For this review, take the finished solid that the model builds, in its own axes (mm). A direction names the side the tool comes from. Round coordinates to 2 decimals unless told otherwise and drop trailing zeros. Loops run counter-clockwise (first coordinate to the right, second up) from the corner with the lowest first, then second, coordinate; pieces in that order, holes last. Notation, with made-up numbers: (19.5, -37) -> (46.5, -37) arc R28 ccw to (46.5, -6) -> close; hole circle Ø7 at (88, -18.75). An arc over 180 degrees is marked (long way). One line per question, with ' | ' between items. Start each with the question number.
1. Consider section D-D (y = 8.5). Write out the cut boundary in (x, z).
2. For faces 1 (the face through (12.52, 11.04, 26.51)), 2 (the face through (13, 10, 60.198)), list the 3-axis set-ups (+Z, -Z, +X, -X, +Y, -Y) from which the entire face can be reached by the end or side of a thin tool; tool diameter is ignored.
3. Consider section C-C (y = 4). Write out the cut boundary in (x, z), and give its area (3 significant figures).
4. Wall thickness on line 1 along Z through (x, y) = (13.75, 13); line 2 along Z through (x, y) = (12, 7.25); line 3 along Z through (x, y) = (20.25, 16.5): over which ranges is each line inside the solid? List them lowest first.
5. Consider section B-B (x = 21). Write out the cut boundary in (y, z) (3 decimals).
6. Consider section A-A (z = 63.5). Write out the cut boundary in (x, y), and give its area (3 significant figures).
7. Draft analysis for pull direction X (two halves, no side actions). For faces 3 (the face through (25.4, 9, 38)), 4 (the face through (3.05, 9.66, 38.03)), 5 (the face through (12.522, 10.478, 49.364)), 6 (the face through (22.35, 9.66, 63.57)), state which applies: pulls with the +X half, pulls with the -X half, needs draft (parallel to the pull), parting line crosses it, or undercut.
Autodesk Inventor part; units mm, degrees
ref_plane "YZ Plane" through (0, 0, 0) normal (1, 0, 0) x (0, 1, 0)
ref_plane "XZ Plane" through (0, 0, 0) normal (0, 1, 0) x (-1, 0, 0)
ref_plane "XY Plane" through (0, 0, 0) normal (0, 0, 1) x (1, 0, 0)
sketch "Sketch1" plane through (0, 0, 0) normal (0, 0, 1) x (1, 0, 0)
  line L0 (0, 0) -> (25.4, 0)
  line L1 (25.4, 0) -> (25.4, 19.05)
  line L2 (25.4, 19.05) -> (0, 19.05)
  line L3 (0, 19.05) -> (0, 0)
  dimension "d0" = 25.4
  dimension "d1" = 19.05
extrude "Stock Bar" add sketch "Sketch1" along normal blind 76.2
sketch "Sketch2" plane through (25.4, 0, 0) normal (1, 0, 0) x (0, 0, -1)
  line L0 (0, 0) -> (0, 19.05)
  line L1 (0, 19.05) -> (-76.2, 19.05)
  point P0 (-51.6636, 9.525)
  point P1 (-24.5364, 9.525)
  dimension "d4" = 27.1272
  dimension "d6" = 9.525
  dimension "d7" = 9.525
  dimension "d29" = 24.5364
hole "Motor Support Mounting Holes" at (25.4, 9.525, 51.6636) at (25.4, 9.525, 24.5364) direction (-1, 0, 0) diameter 4.9784 end up to surface
sketch "Sketch3" plane through (0, 19.05, 0) normal (0, 1, 0) x (1, 0, 0)
  line L0 (6.35, -12.7) -> (19.05, -12.7) construction
  line L1 (6.35, -16.002) -> (19.05, -16.002)
  line L2 (19.05, -9.398) -> (6.35, -9.398)
  arc A0 (6.35, -9.398) -> (6.35, -16.002) centre (6.35, -12.7) ccw
  arc A1 (19.05, -16.002) -> (19.05, -9.398) centre (19.05, -12.7) ccw
  line L3 (6.35, -63.5) -> (19.05, -63.5) construction
  line L4 (6.35, -66.802) -> (19.05, -66.802)
  line L5 (19.05, -60.198) -> (6.35, -60.198)
  arc A2 (6.35, -60.198) -> (6.35, -66.802) centre (6.35, -63.5) ccw
  arc A3 (19.05, -66.802) -> (19.05, -60.198) centre (19.05, -63.5) ccw
  line L6 (6.35, -38.1) -> (19.05, -38.1) construction
  line L7 (6.35, -41.402) -> (19.05, -41.402)
  line L8 (19.05, -34.798) -> (6.35, -34.798)
  arc A4 (6.35, -34.798) -> (6.35, -41.402) centre (6.35, -38.1) ccw
  arc A5 (19.05, -41.402) -> (19.05, -34.798) centre (19.05, -38.1) ccw
  line L9 (25.4, 0) -> (25.4, -76.2)
  line L10 (25.4, -76.2) -> (0, -76.2)
  point P0 (12.7, -12.7)
  point P1 (12.7, -63.5)
  point P2 (12.7, -38.1)
  dimension "d15" = 3.302
  dimension "d16" = 3.302
  dimension "d17" = 3.302
  dimension "d18" = 12.7
  dimension "d19" = 12.7
  dimension "d20" = 12.7
  dimension "d21" = 25.4
  dimension "d22" = 25.4
  dimension "d23" = 6.35
  dimension "d24" = 6.35
  dimension "d25" = 6.35
  dimension "d26" = 12.7
extrude "Table Mounting Slots" cut sketch "Sketch3" against normal blind 101.6
properties part number "Motor Base" material "Aluminum 6061"
Answer block:
1) outline: (0, 0) -> (25.4, 0) -> (25.4, 22.27) -> (0, 22.27) -> close; (0, 26.8) -> (25.4, 26.8) -> (25.4, 49.4) -> (0, 49.4) -> close; (0, 53.93) -> (25.4, 53.93) -> (25.4, 76.2) -> (0, 76.2) -> close; hole (6.35, 9.4) -> (19.05, 9.4) arc R3.3 ccw to (19.05, 16) -> (6.35, 16) arc R3.3 ccw to start; hole (6.35, 34.8) -> (19.05, 34.8) arc R3.3 ccw to (19.05, 41.4) -> (6.35, 41.4) arc R3.3 ccw to start; hole (6.35, 60.2) -> (19.05, 60.2) arc R3.3 ccw to (19.05, 66.8) -> (6.35, 66.8) arc R3.3 ccw to start
2) face 1: +X, -X | face 2: +Y, -Y
3) outline: (0, 0) -> (25.4, 0) -> (25.4, 76.2) -> (0, 76.2) -> close; hole (6.35, 9.4) -> (19.05, 9.4) arc R3.3 ccw to (19.05, 16) -> (6.35, 16) arc R3.3 ccw to start; hole (6.35, 34.8) -> (19.05, 34.8) arc R3.3 ccw to (19.05, 41.4) -> (6.35, 41.4) arc R3.3 ccw to start; hole (6.35, 60.2) -> (19.05, 60.2) arc R3.3 ccw to (19.05, 66.8) -> (6.35, 66.8) arc R3.3 ccw to start | area: 1,580 mm2
4) line 1: z = 0 to 9.4, 16 to 34.8, 41.4 to 60.2, 66.8 to 76.2 | line 2: z = 0 to 9.4, 16 to 23.53, 25.55 to 34.8, 41.4 to 50.65, 52.67 to 60.2, 66.8 to 76.2 | line 3: z = 0 to 9.62, 15.78 to 35.02, 41.18 to 60.42, 66.58 to 76.2
5) outline: (0, 0) -> (19.05, 0) -> (19.05, 10.035) -> (0, 10.035) -> close; (0, 15.365) -> (19.05, 15.365) -> (19.05, 35.435) -> (0, 35.435) -> close; (0, 40.765) -> (19.05, 40.765) -> (19.05, 60.835) -> (0, 60.835) -> close; (0, 66.165) -> (19.05, 66.165) -> (19.05, 76.2) -> (0, 76.2) -> close; hole circle Ø4.978 at (9.525, 24.536); hole circle Ø4.978 at (9.525, 51.664)
6) outline: (0, 0) -> (3.05, 0) -> (3.05, 19.05) -> (0, 19.05) -> close; (22.35, 0) -> (25.4, 0) -> (25.4, 19.05) -> (22.35, 19.05) -> close | area: 116 mm2
7) face 3: pulls with the +X half | face 4: undercut | face 5: needs draft | face 6: undercut
